from build123d import *

# Parameters (mm, degrees)
ESBO_O1_R                = 5
ESBO_O1_R_2              = 2.65
RESSALTO_EXTRUS_O3_DEPTH = 7
RESSALTO_EXTRUS_O4_START = -20
ESBO_O3_W                = 10
ESBO_O3_H                = 6.5
RESSALTO_EXTRUS_O4_DEPTH = 5
CORTE_EXTRUS_O2_DEPTH    = 8
ESBO_O6_R                = 1.65
CORTE_EXTRUS_O3_DEPTH    = 17
CORTE_EXTRUS_O4_DEPTH    = 4
CHANFRO1_SIZE            = 2.5
CORTE_EXTRUS_O1_DEPTH    = 2
CHANFRO2_SIZE            = 0.5


with BuildPart() as part:
    # Esboço1 → Ressalto-extrusão3 (new body)
    with BuildSketch(Plane.XY):
        with BuildLine():
            Line((7.982953463, 0.015906926), (7.982953463, -37.484093074))
            ThreePointArc((7.982953463, -37.484093074), (6.518487369, -41.01962698), (2.982953463, -42.484093074))
            Line((2.982953463, -42.484093074), (-3.017046537, -42.484093074))
            ThreePointArc((-3.017046537, -42.484093074), (-6.552580443, -41.01962698), (-8.017046537, -37.484093074))
            Line((-8.017046537, -37.484093074), (-8.017046537, 0.015906926))
            ThreePointArc((-8.017046537, 0.015906926), (-0.017046537, 8.015906926), (7.982953463, 0.015906926))
        make_face()
        with Locations((-0.017046537, 0.015906926)):
            Circle(ESBO_O1_R, mode=Mode.SUBTRACT)
        with Locations((-0.017046537, -32.484093074)):
            Circle(ESBO_O1_R_2, mode=Mode.SUBTRACT)
    extrude(amount=RESSALTO_EXTRUS_O3_DEPTH)

    # Esboço3 → Ressalto-extrusão4 (add)
    with BuildSketch(Plane.XZ.offset(42.484093074).offset(RESSALTO_EXTRUS_O4_START)):
        with BuildLine():
            Line((7.982953463, 0), (-8.017046537, 0))
            Line((-8.017046537, 0), (-8.017046537, -15))
            ThreePointArc((-8.017046537, -15), (-6.552580443, -18.535533906), (-3.017046537, -20))
            Line((-3.017046537, -20), (2.982953463, -20))
            ThreePointArc((2.982953463, -20), (6.518487369, -18.535533906), (7.982953463, -15))
            Line((7.982953463, -15), (7.982953463, 0))
        make_face()
        with Locations((-0.017046537, -10)):
            Rectangle(ESBO_O3_W, ESBO_O3_H, mode=Mode.SUBTRACT)
    extrude(amount=-RESSALTO_EXTRUS_O4_DEPTH)

    # Esboço5 → Corte-extrusão2 (cut, through all)
    with BuildSketch(Plane(origin=(0, 0, 0), x_dir=(-1, 0, 0), z_dir=(0, 0, -1))):
        with BuildLine():
            Line((-4.482953463, -2.163542545), (-4.482953463, -16.484093074))
            Line((-4.482953463, -16.484093074), (-7.982953463, -16.484093074))
            Line((-7.982953463, -16.484093074), (-7.982953463, -17.484093074))
            Line((-7.982953463, -17.484093074), (-3.482953463, -17.484093074))
            Line((-3.482953463, -17.484093074), (-3.482953463, -3.554807288))
            ThreePointArc((-3.482953463, -3.554807288), (-4.04299095, -2.902328089), (-4.482953463, -2.163542545))
        make_face()
    extrude(amount=-CORTE_EXTRUS_O2_DEPTH, mode=Mode.SUBTRACT)

    # Esboço6 → Corte-extrusão3 (cut, through all)
    with BuildSketch(Plane(origin=(7.982953463, 0, 0), x_dir=(0, 0, -1), z_dir=(1, 0, 0))):
        with Locations((-3.5, -9.484093074)):
            Circle(ESBO_O6_R)
    extrude(amount=-CORTE_EXTRUS_O3_DEPTH, mode=Mode.SUBTRACT)

    # Esboço7 → Corte-extrusão4 (cut)
    with BuildSketch(Plane(origin=(-8.017046537, 0, 0), x_dir=(0, 0, -1), z_dir=(1, 0, 0))):
        Polygon((-6.3, -7.86751232), (-6.3, -11.100673827), (-3.5, -12.717254581), (-0.7, -11.100673827), (-0.7, -7.86751232), (-3.5, -6.250931566), align=None)
    extrude(amount=CORTE_EXTRUS_O4_DEPTH, mode=Mode.SUBTRACT)

    # Chanfro1
    chanfro1_edges = [part.edges().sort_by_distance(p)[0] for p in [
        (-2.267046537, -17.484093074, 0),
    ]]
    chamfer(chanfro1_edges, length=CHANFRO1_SIZE)

    # Esboço4 → Corte-extrusão1 (cut)
    with BuildSketch(Plane(origin=(0, 0, 0), x_dir=(-1, 0, 0), z_dir=(0, 0, -1))):
        with BuildLine():
            Line((-2.982953463, -42.484093074), (3.017046537, -42.484093074))
            ThreePointArc((3.017046537, -42.484093074), (6.552580443, -41.01962698), (8.017046537, -37.484093074))
            Line((8.017046537, -37.484093074), (8.017046537, -22.484093074))
            Line((8.017046537, -22.484093074), (-7.982953463, -22.484093074))
            Line((-7.982953463, -22.484093074), (-7.982953463, -37.484093074))
            ThreePointArc((-7.982953463, -37.484093074), (-6.518487369, -41.01962698), (-2.982953463, -42.484093074))
        make_face()
    extrude(amount=-CORTE_EXTRUS_O1_DEPTH, mode=Mode.SUBTRACT)

    # Chanfro2
    chanfro2_edges = [part.edges().sort_by_distance(p)[0] for p in [
        (-2.667046537, -32.484093074, 7),
        (4.482953463, -9.323817809, 7),
        (-4.077084024, 2.934141942, 7),
        (3.482953463, -10.519450181, 7),
        (5.732953463, -17.484093074, 7),
        (7.982953463, -27.484093074, 7),
        (6.518487369, -41.01962698, 7),
        (-0.017046537, -42.484093074, 7),
        (-6.552580443, -41.01962698, 7),
        (-8.017046537, -18.734093074, 7),
        (-0.017046537, 8.015906926, 7),
        (6.232953463, -16.484093074, 7),
    ]]
    chamfer(chanfro2_edges, length=CHANFRO2_SIZE)


solid = part.part
For this review, take the finished solid that the model builds, in its own axes (mm). A direction names the side the tool comes from. Round coordinates to 2 decimals unless told otherwise and drop trailing zeros. Write each loop counter-clockwise with the first axis right and the second up, starting at its lowest first coordinate (ties: lowest second). Pieces come first, ordered by that corner, then holes. Notation, with made-up numbers: (-3.75, 65) - (17.25, 65) arc R15 ccw to (17.25, 71) - close; hole circle Ø11 at (23.25, 86.5). An arc over 180 degrees is marked (long way). Write item = value, one per line. Start each with the question number.
1. Wall thickness on L1, parallel to Y at x = 5.35, z = 3.5; L2, parallel to Y at x = 1, z = 3.5; L3, parallel to X at y = -8, z = 5: over which ranges is each line inside the solid? List them lowest first.
2. Consider section D-D on z = -4.5. State the section outline as (x, y) points, plus the area to 3 significant figures.
3. Consider section A-A on z = -9. State the section outline as (x, y) points.
4. Draft analysis for pull direction Y (two halves, no side actions). For faces 1 (the face through (-0.215, -7.848, 3.715)), 2 (the face through (6.479, -20.019, -18.574)), 3 (the face through (-0.193, 8.014, 3.204)), 4 (the face through (6.56, -40.98, 4.22)), state which applies: released by +Y, released by -Y, zero draft, split by the parting line, or undercut.
5. Consider section B-B on y = -20.5. State the section outline as (x, z) points, plus the area to 3 significant figures.
6. Consider section C-C on x = -1.25. Give the number of separate pieces and of enclosed holes in the cut face, plus the area to 3 significant figures.
7. For pin 1 Ø4 at (x, z) = (6.5, 4.5) entering from -Y; pin 2 Ø8 at (x, z) = (3.5, -5.5) entering from +Y; pin 3 Ø8 at (x, y) = (1, -37) entering from -Z; pin 4 Ø3 at (y, z) = (-9.48, 3.5) entering from -X, all flat-tipped, find the tip position at first contact; note any pin that passes through.
8. For faces 5 (the face through (-6.045, -7.048, 4.88)), 6 (the face through (4.983, -20, -10)), 7 (the face through (-2.187, -16.252, -1.268)), 8 (the face through (6, -16.484, 3)), list the 3-axis set-ups (+Z, -Z, +X, -X, +Y, -Y) from which the entire face can be reached by the end or side of a thin tool; tool diameter is ignored.
Evaluation:
q1.L1 = -41.89 to -17.48, -16.48 to -11.13, -7.83 to 5.95
q1.L2 = -42.48 to -34.93, -30.04 to -11.13, -7.83 to -4.88, 4.91 to 7.95
q1.L3 = -4.02 to 3.48, 4.48 to 7.98
q2.outline = (-8.02, -22.48) - (7.98, -22.48) - (7.98, -17.48) - (-8.02, -17.48) - close
q2.area = 80.0 mm2
q3.outline = (-8.02, -22.48) - (-5.02, -22.48) - (-5.02, -17.48) - (-8.02, -17.48) - close; (4.98, -22.48) - (7.98, -22.48) - (7.98, -17.48) - (4.98, -17.48) - close
q4.face_1 = undercut
q4.face_2 = zero draft
q4.face_3 = released by +Y
q4.face_4 = released by -Y
q5.outline = (-8.02, -15) arc R5 ccw to (-3.02, -20) - (2.98, -20) arc R5 ccw to (7.98, -15) - (7.98, 6.5) - (7.48, 7) - (-7.52, 7) - (-8.02, 6.5) - close; hole (-5.02, -13.25) - (4.98, -13.25) - (4.98, -6.75) - (-5.02, -6.75) - close
q5.area = 356 mm2
q6.separate_pieces = 4
q6.enclosed_holes = 1
q6.area = 283 mm2
q7.pin_1 = -42.25
q7.pin_2 = -16.48
q7.pin_3 = 2
q7.pin_4 = through
q8.face_5 = -X
q8.face_6 = +Y, -Y
q8.face_7 = -Z, +X, -X, +Y
q8.face_8 = +Z, -Z, +X
